Can you work these out from the drawing? Everything is in mm from the part's minimum corner. Round coordinates to 2 decimals unless told otherwise and drop trailing zeros. Loops run counter-clockwise (first coordinate to the right, second up) from the corner with the lowest first, then second, coordinate; pieces in that order, holes last. Notation, with made-up numbers: (77, 68.25) - (83, 68.25) arc R11 cw to (83, 81.25) - close; hole circle Ø10 at (41, -3). An arc over 180 degrees is marked (long way). Return JSON: item names as keys, results as strings. Group by question number.
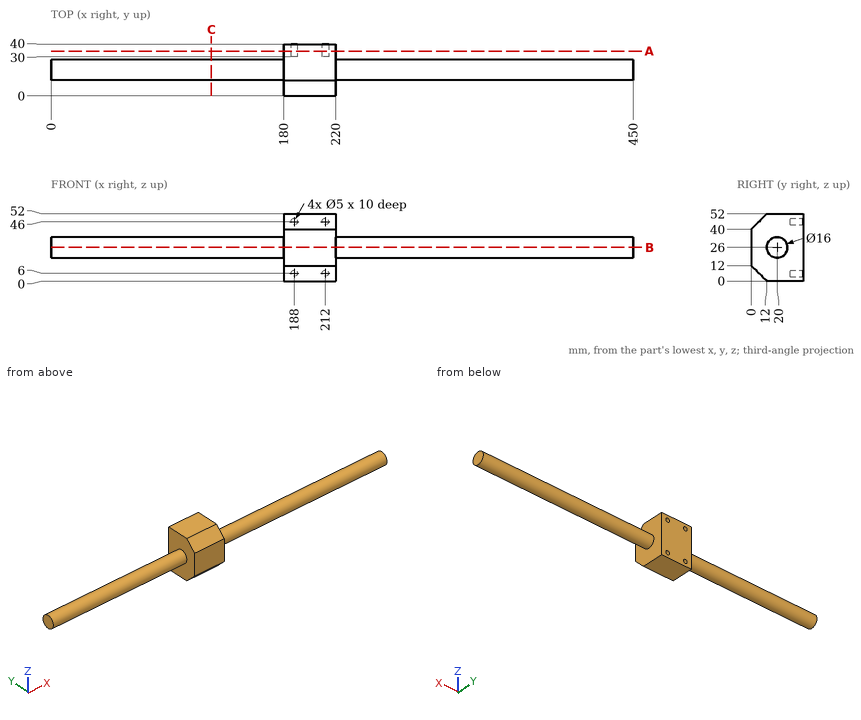
Q1. Imagine slicing it at C-C, the plane x = 124. List the corners of the cut face in (y, z) for me, and give its area (3 significant figures).
Q2. Please list where these lines run through material, in increasing order: line 1 (Z direction, x = 188, y = 36.5); line 2 (X direction, y = 31.5, z = 26); line 3 (Z direction, x = 157.5, y = 21).
Q3. Will these pins go through, and if not, where does the flat tip stop? pin 1 Ø5 at (x, z) = (245.5, 34) entering from -Y; pin 2 Ø3 at (x, z) = (188, 6) entering from -Y; pin 3 Ø1.5 at (y, z) = (35.5, 27) entering from -X; pin 4 Ø6 at (x, y) = (156.5, 7) entering from -Z.
Q4. Imagine slicing it at A-A, the plane y = 34.5. List the corners of the cut face in (x, z) for me.
Q5. Imagine slicing it at B-B, the plane z = 26. List the corners of the cut face in (x, y) for me, and give its area (3 significant figures).
Output values:
{
 "1": {"outline": "circle Ø16 at (20, 26)", "area": "201 mm^2"},
 "2": {"line 1": "z = 0 to 3.5, 8.5 to 43.5, 48.5 to 52", "line 2": "x = 180 to 220", "line 3": "z = 18.06 to 33.94"},
 "3": {"pin 1": "stops at y = 14.19", "pin 2": "stops at y = 4.5", "pin 3": "stops at x = 180", "pin 4": "passes through"},
 "4": {"outline": "(180, 0) - (220, 0) - (220, 52) - (180, 52) - close; hole circle Ø5 at (188, 6); hole circle Ø5 at (188, 46); hole circle Ø5 at (212, 6); hole circle Ø5 at (212, 46)"},
 "5": {"outline": "(0, 12) - (180, 12) - (180, 0) - (220, 0) - (220, 12) - (450, 12) - (450, 28) - (220, 28) - (220, 40) - (180, 40) - (180, 28) - (0, 28) - close", "area": "8,160 mm^2"}
}
